Study the drawing (mm; zero at the part's minimum x, y, z) and answer. Round coordinates to 2 decimals unless told otherwise and drop trailing zeros. Write each loop counter-clockwise with the first axis right and the second up, starting at its lowest first coordinate (ties: lowest second). Pieces come first, ordered by that corner, then holes.
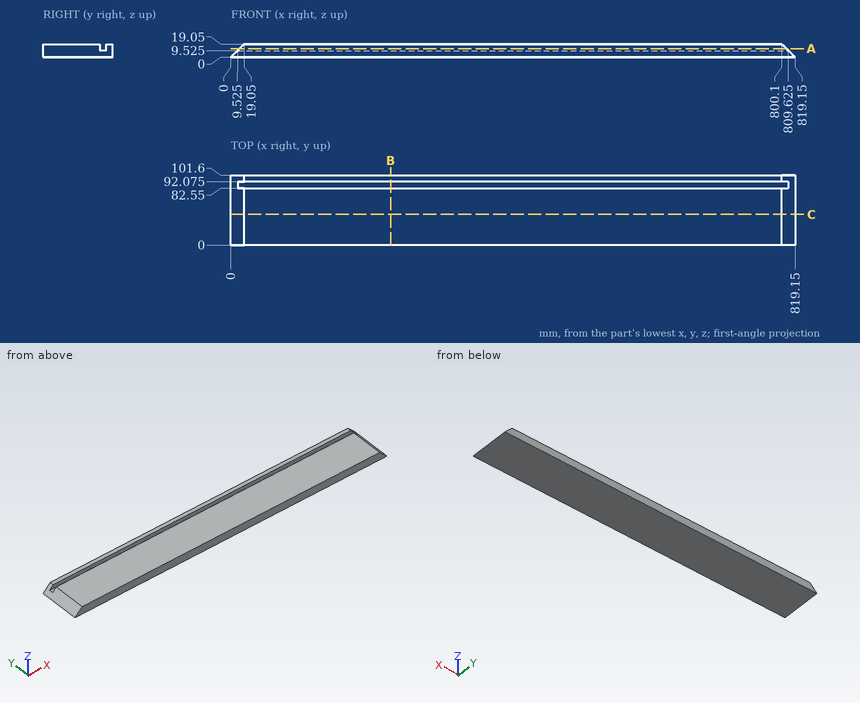
Q1. Find section C-C (y = 44.5). Determine the outline of the cut face in (x, z).
Q2. Given pin 1 (2 mm diameter, centred on y = 57, z = 7, fed in from +X); pin 2 (5 mm diameter, centred on y = 43.5, z = 4, fed in from +X); pin 3 (1 mm diameter, centred on y = 71.5, z = 7.5, fed in from -X), each flat-ended and moving along its own axis, determine where each tip first touches the part or whether it passes through.
Q3. Find section B-B (x = 232). Determine the outline of the cut face in (y, z) (3 decimals), plus the area to 3 significant figures.
Q4. Find section A-A (z = 12.5). Determine the outline of the cut face in (x, y) (3 decimals), plus the area to 3 significant figures.
Q5. Find the intervals of material crossed by L1, parallel to Y at x = 108, z = 16.5 (3 decimals); L2, parallel to Z at x = 666.5, y = 87 (3 decimals); L3, parallel to X at y = 41, z = 15.5, in increasing order.
Report:
1. outline: (0, 0) - (819.15, 0) - (800.1, 19.05) - (19.05, 19.05) - close
2. pin 1: stops at x = 813.15
2. pin 2: stops at x = 817.65
2. pin 3: stops at x = 7
3. outline: (0, 0) - (101.6, 0) - (101.6, 19.05) - (92.075, 19.05) - (92.075, 9.525) - (82.55, 9.525) - (82.55, 19.05) - (0, 19.05) - close
3. area: 1,840 mm2
4. outline: (12.5, 0) - (806.65, 0) - (806.65, 82.55) - (12.5, 82.55) - close; (12.5, 92.075) - (806.65, 92.075) - (806.65, 101.6) - (12.5, 101.6) - close
4. area: 73,100 mm2
5. L1: y = 0 to 82.55, 92.075 to 101.6
5. L2: z = 0 to 9.525
5. L3: x = 15.5 to 803.65
